Geometry check sheet. Reference: the model listing, model coordinates, mm. Coordinates: 2 decimals unless noted, no trailing zeros. Write each loop counter-clockwise with the first axis right and the second up, starting at its lowest first coordinate (ties: lowest second). Pieces come first, ordered by that corner, then holes. Notation, with made-up numbers: (-34.75, 66) -> (-21.75, 66) arc R21 ccw to (-21.75, 89) -> close; hole circle Ø6 at (70.5, 80). An arc over 180 degrees is marked (long way). Put each result on its own line as item: value. Start each with the question number.
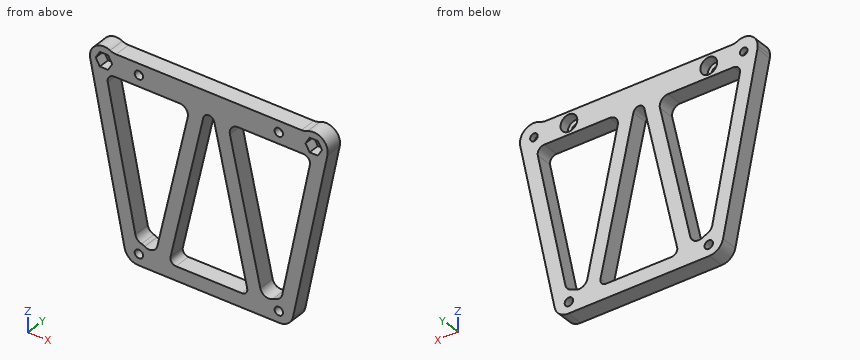
from build123d import *

# Parameters (mm, degrees)
SKETCH_2_R          = 1.5
SKETCH_2_R_2        = 1.35
EXTRUDE_1_DEPTH     = 6
SKETCH_5_R          = 3
CUT_EXTRUDE_4_DEPTH = 3.5
CUT_EXTRUDE_5_DEPTH = 4
CUT_EXTRUDE_6_DEPTH = 7


with BuildPart() as part:
    # 草图2 → 凸台-拉伸1 (new body)
    with BuildSketch(Plane(origin=(0, 0, 0), x_dir=(1, 0, 0), z_dir=(0, 1, 0))):
        with BuildLine():
            Line((-42.5, -62), (-42.5, 1))
            ThreePointArc((-42.5, 1), (-41.621320344, 3.121320344), (-39.5, 4))
            Line((-39.5, 4), (39.5, 4))
            ThreePointArc((39.5, 4), (41.621320344, 3.121320344), (42.5, 1))
            Line((42.5, 1), (42.5, -62))
            ThreePointArc((42.5, -62), (40.155442773, -66.236581603), (35.320550528, -66.5))
            ThreePointArc((35.320550528, -66.5), (34.259135045, -66.126602828), (33.141101056, -66))
            Line((33.141101056, -66), (-33.141101056, -66))
            ThreePointArc((-33.141101056, -66), (-34.259135045, -66.126602828), (-35.320550528, -66.5))
            ThreePointArc((-35.320550528, -66.5), (-40.155442773, -66.236581603), (-42.5, -62))
        make_face()
        with Locations((-25, 0)):
            Circle(SKETCH_2_R, mode=Mode.SUBTRACT)
        with Locations((25, 0)):
            Circle(SKETCH_2_R, mode=Mode.SUBTRACT)
        with Locations((-25, -62)):
            Circle(SKETCH_2_R, mode=Mode.SUBTRACT)
        with Locations((25, -62)):
            Circle(SKETCH_2_R, mode=Mode.SUBTRACT)
        with Locations((-37.5, -62)):
            Circle(SKETCH_2_R_2, mode=Mode.SUBTRACT)
        with Locations((37.5, -62)):
            Circle(SKETCH_2_R_2, mode=Mode.SUBTRACT)
    extrude(amount=EXTRUDE_1_DEPTH)

    # 草图5 → 切除-拉伸4 (cut)
    with BuildSketch(Plane(origin=(0, 6, 0), x_dir=(1, 0, 0), z_dir=(0, 1, 0))):
        with Locations((-25, -62)):
            Circle(SKETCH_5_R)
        with Locations((25, -62)):
            Circle(SKETCH_5_R)
    extrude(amount=-CUT_EXTRUDE_4_DEPTH, mode=Mode.SUBTRACT)

    # 草图6 → 切除-拉伸5 (cut)
    with BuildSketch(Plane.XZ):
        Polygon((-36.027756814, 64.55), (-38.972243186, 64.55), (-40.444486373, 62), (-38.972243186, 59.45), (-36.027756814, 59.45), (-34.555513627, 62), align=None)
        Polygon((34.555513627, 62), (36.027756814, 64.55), (38.972243186, 64.55), (40.444486373, 62), (38.972243186, 59.45), (36.027756814, 59.45), align=None)
    extrude(amount=-CUT_EXTRUDE_5_DEPTH, mode=Mode.SUBTRACT)

    # 草图7 → 切除-拉伸6 (cut, through all)
    with BuildSketch(Plane(origin=(0, 6, 0), x_dir=(1, 0, 0), z_dir=(0, 1, 0))):
        with BuildLine():
            Line((-33.791892668, -58), (-10.464489806, -58))
            ThreePointArc((-10.464489806, -58), (-8.124836357, -56.877770417), (-7.535601784, -54.350681158))
            Line((-7.535601784, -54.350681158), (-18.406585082, -5.314844354))
            ThreePointArc((-18.406585082, -5.314844354), (-20.164908448, -3.201957847), (-22.905984631, -3.408093255))
            ThreePointArc((-22.905984631, -3.408093255), (-23.45168362, -3.688186057), (-24.033791208, -3.88155131))
            ThreePointArc((-24.033791208, -3.88155131), (-25.477663554, -4.719677831), (-26.249960939, -6.199806259))
            Line((-26.249960939, -6.199806259), (-36.120076242, -55.155578159))
            ThreePointArc((-36.120076242, -55.155578159), (-35.629770137, -57.129288416), (-33.791892668, -58))
        make_face()
        with BuildLine():
            Line((-13.702409134, -3.432879228), (-1.952592014, -56.432879228))
            ThreePointArc((-1.952592014, -56.432879228), (0, -58), (1.952592014, -56.432879228))
            Line((1.952592014, -56.432879228), (13.702409134, -3.432879228))
            ThreePointArc((13.702409134, -3.432879228), (13.309586086, -1.748153056), (11.74981712, -1))
            Line((11.74981712, -1), (-11.74981712, -1))
            ThreePointArc((-11.74981712, -1), (-13.309586086, -1.748153056), (-13.702409134, -3.432879228))
        make_face()
        with BuildLine():
            Line((18.406585082, -5.314844354), (7.535601784, -54.350681158))
            ThreePointArc((7.535601784, -54.350681158), (8.124836357, -56.877770417), (10.464489806, -58))
            Line((10.464489806, -58), (33.791892668, -58))
            ThreePointArc((33.791892668, -58), (35.629770137, -57.129288416), (36.120076242, -55.155578159))
            Line((36.120076242, -55.155578159), (26.249960939, -6.199806259))
            ThreePointArc((26.249960939, -6.199806259), (25.477663554, -4.719677831), (24.033791208, -3.88155131))
            ThreePointArc((24.033791208, -3.88155131), (23.45168362, -3.688186057), (22.905984631, -3.408093255))
            ThreePointArc((22.905984631, -3.408093255), (20.164908448, -3.201957847), (18.406585082, -5.314844354))
        make_face()
        with BuildLine():
            Line((-42.401377208, -61.011819111), (-30.102990111, -0.011819111))
            ThreePointArc((-30.102990111, -0.011819111), (-28.368559031, 2.869166864), (-25.201612903, 4))
            Line((-25.201612903, 4), (-42.5, 4))
            Line((-42.5, 4), (-42.5, -62))
            ThreePointArc((-42.5, -62), (-42.47528321, -61.503454956), (-42.401377208, -61.011819111))
        make_face()
        with BuildLine():
            Line((42.401377208, -61.011819111), (30.102990111, -0.011819111))
            ThreePointArc((30.102990111, -0.011819111), (28.368559031, 2.869166864), (25.201612903, 4))
            Line((25.201612903, 4), (42.5, 4))
            Line((42.5, 4), (42.5, -62))
            ThreePointArc((42.5, -62), (42.47528321, -61.503454956), (42.401377208, -61.011819111))
        make_face()
    extrude(amount=-CUT_EXTRUDE_6_DEPTH, mode=Mode.SUBTRACT)


solid = part.part
Item 1: Section check A-A, the plane x = 4. Enter the section's corners in (y, z), and give its area (3 significant figures).
Item 2: Scan lines: line 1 along X through (y, z) = (4.55, 62); line 2 along X through (y, z) = (2.4, 0); line 3 along X through (y, z) = (0.9, 62). Record each from-to range of solid material in increasing order. Write a range as [from, to].
Item 3: Section check C-C, the plane z = 28.5. Enter the section's corners in (x, y), and give its area (3 significant figures).
Item 4: Go/stop test with flat-tipped pins: P1, Ø2, axis at y = 2, z = 28.5, coming from the -X side; P2, Ø1.8, axis at x = -24, z = 61, coming from the +Y side; P3, Ø3.5, axis at x = 37.5, z = 62, coming from the -Y side. Record where each tip stops, or that it passes through.
Item 5: Section check B-B, the plane y = 5. Give the number of separate pieces and of enclosed holes in the cut face, and give its area (3 significant figures).
From the geometry:
1. outline: (0, -4) -> (6, -4) -> (6, 1) -> (0, 1) -> close; (0, 47.2) -> (6, 47.2) -> (6, 66) -> (0, 66) -> close
1. area: 143 mm²
2. line 1: [-42.5, -38.85], [-36.15, -28], [-22, 22], [28, 36.15], [38.85, 42.5]
2. line 2: [-30.1, -26.5], [-23.5, 23.5], [26.5, 30.1]
2. line 3: [-42.5, -40.44], [-34.56, -26.5], [-23.5, 23.5], [26.5, 34.56], [40.44, 42.5]
3. outline: (-35.85, 0) -> (-30.75, 0) -> (-30.75, 6) -> (-35.85, 6) -> close; (-13.27, 0) -> (-8.15, 0) -> (-8.15, 6) -> (-13.27, 6) -> close; (8.15, 0) -> (13.27, 0) -> (13.27, 6) -> (8.15, 6) -> close; (30.75, 0) -> (35.85, 0) -> (35.85, 6) -> (30.75, 6) -> close
3. area: 123 mm²
4. P1: x = -36.05
4. P2: y = 2.5
4. P3: y = 4
5. separate pieces: 1
5. enclosed holes: 9
5. area: 2,100 mm²
